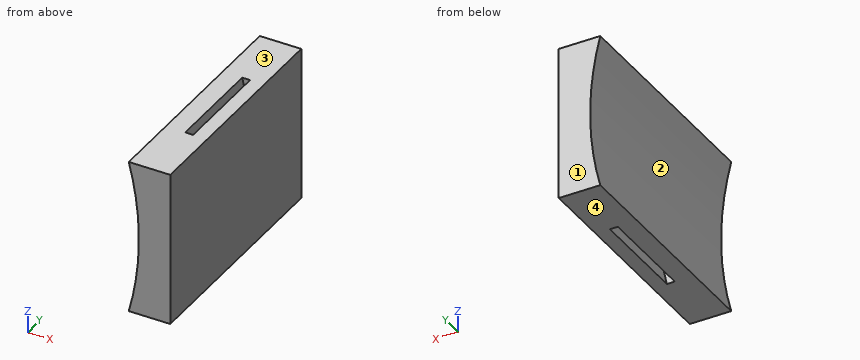
Autodesk Inventor part; units mm, degrees
ref_plane "YZ Plane" through (0, 0, 0) normal (1, 0, 0) x (0, 1, 0)
ref_plane "XZ Plane" through (0, 0, 0) normal (0, 1, 0) x (-1, 0, 0)
ref_plane "XY Plane" through (0, 0, 0) normal (0, 0, 1) x (1, 0, 0)
sketch "Sketch1" plane through (0, 0, 0) normal (0, 1, 0) x (-1, 0, 0)
  line L0 (0, 20.193) -> (0, -20.193)
  line L1 (0, -20.193) -> (3.6912, -20.193)
  line L2 (0, 20.193) -> (3.6912, 20.193)
  arc A0 (10.8286, 20.193) -> (10.8286, -20.193) centre (86.8455, 0) ccw
  arc A1 (5.7486, 20.193) -> (5.7486, -20.193) centre (86.8455, 0) ccw
  arc A2 (3.6912, 20.193) -> (3.6912, -20.193) centre (86.8455, 0) ccw
  line L3 (5.7486, 20.193) -> (10.8286, 20.193)
  line L4 (3.6912, 20.193) -> (5.7486, 20.193)
  line L5 (3.6912, -20.193) -> (5.7486, -20.193)
  line L6 (5.7486, -20.193) -> (10.8286, -20.193)
  point P0 (0, 0)
  point P1 (8.1923, 0)
  point P2 (0, 0)
  dimension "d0" = 2.0574
  dimension "d1" = 5.08
  dimension "d2" = 8.1923
  dimension "d3" = 40.386
  dimension "d4" = 10.8286
extrude "Extrusion1" add sketch "Sketch1" along normal mid plane 60.1218
extrude "Extrusion2" cut sketch "Sketch1" along normal mid plane 26.162 contours L4 A1 L5 A2
equation "\"d4\" = Height"
properties part number "Cover" material "Glass"
For this review, take the finished solid that the model builds, in its own axes (mm). Face numbers are marked on the shaded views. Give positions to 0.01 mm unless a question says otherwise; leave off trailing zeros. Write each loop counter-clockwise with the first axis right and the second up, starting at its lowest first coordinate (ties: lowest second). Pieces come first, ordered by that corner, then holes. Notation, with made-up numbers: M 47,-28.5 L 54,-28.5 A24 ccw 54,-3.5 Z; hole C 32,79.5 d1. An arc over 180 degrees is marked long. Answer as a JSON object with one key per item and string values. Group by question number.
Item 1: Consider section A-A on y = 7. Write out the cut boundary in (x, z), plus the area to 3 significant figures.
Item 2: Consider section D-D on x = -4.75. Write out the cut boundary in (y, z).
Item 3: Consider section C-C on y = 26. Write out the cut boundary in (x, z).
Item 4: For pin 1 Ø8 at (y, z) = (2, -9.5) entering from -X; pin 2 Ø10 at (y, z) = (-22, -12) entering from -X, all flat-tipped, find the tip position at first contact; note any pin that passes through.
Item 5: Draft analysis for pull direction Z (two halves, no side actions). For the marked faces 1, 2, 3 and 4, state which applies: +Z half, -Z half, draft (parallel to the pull), parting line (faces both ways), or undercut.
Item 6: Consider section B-B on z = 14. Write out the cut boundary in (x, y), plus the area to 3 significant figures.
Item 7: For probe 1 along Y at (x, z) = (-3.5, -14.5); probe 2 along X at (y, z) = (5, -13.5); probe 3 along X at (y, z) = (-3.5, -15), list the stretches that pass through material, from the lowest coordinate up. Write a range as [from, to].
Check result:
{
 "1": {"outline": "M -10.83,-20.19 L -5.75,-20.19 A83.57 ccw -5.75,20.19 L -10.83,20.19 A78.65 cw Z; M -3.69,-20.19 L 0,-20.19 L 0,20.19 L -3.69,20.19 A85.57 cw Z", "area": "285 mm^2"},
 "2": {"outline": "M -30.06,-20.19 L -13.08,-20.19 L -13.08,-15.65 L 13.08,-15.65 L 13.08,-20.19 L 30.06,-20.19 L 30.06,20.19 L 13.08,20.19 L 13.08,15.65 L -13.08,15.65 L -13.08,20.19 L -30.06,20.19 Z"},
 "3": {"outline": "M -10.83,-20.19 L 0,-20.19 L 0,20.19 L -10.83,20.19 A78.65 cw Z"},
 "4": {"pin 1": "stops at x = -9.36", "pin 2": "stops at x = -10.05"},
 "5": {"face 1": "draft", "face 2": "undercut", "face 3": "+Z half", "face 4": "-Z half"},
 "6": {"outline": "M -9.45,-30.06 L 0,-30.06 L 0,30.06 L -9.45,30.06 Z; hole M -4.45,-13.08 L -2.43,-13.08 L -2.43,13.08 L -4.45,13.08 Z", "area": "515 mm^2"},
 "7": {"probe 1": "y = [-30.06, -13.08], [13.08, 30.06]", "probe 2": "x = [-9.36, -4.37], [-2.35, 0]", "probe 3": "x = [-9.64, -4.63], [-2.6, 0]"}
}
